The model under review builds one solid part; all positions refer to its coordinate system, in mm. A direction names the side the tool comes from. Coordinates: 2 decimals unless noted, no trailing zeros. Write each loop counter-clockwise with the first axis right and the second up, starting at its lowest first coordinate (ties: lowest second). Pieces come first, ordered by that corner, then holes.
1) For line 1 (X direction, y = -6, z = 101.5); line 2 (Y direction, x = 39, z = 139); line 3 (X direction, y = 52, z = 13), list the stretches that pass through material, from the lowest coordinate up.
2) Mouldability with a two-part tool opening along X and no side actions: class faces 1 (the flat face through (22, 27, 60)), 2 (the flat face through (0, -2, 81)), 3 (the flat face through (-5, 24, 97)) as released by +X, released by -X, zero draft, split by the parting line, or undercut.
3) Add section D-D, the plane x = 30.5. State the section outline as (y, z) points, then the cut area to 3 significant figures.
4) Add section B-B, the plane y = 40. State the section outline as (x, z) points, then the cut area to 3 significant figures.
5) Machinability: for faces 4 (the flat face through (-44, 0, 81)), 5 (the flat face through (5, 24, 97)), 6 (the flat face through (44, 0, 81)), 7 (the flat face through (-26, -7, 81)), which of the approach directions +Z, -Z, +X, -X, +Y, -Y give a long, thin tool a straight path to every point of the face, cutting with its end or side? Answer none if there is none.
6) Add section C-C, the plane z = 146. State the section outline as (x, y) points, then the cut area to 3 significant figures.
7) For P1, Ø9, axis at x = -18.5, y = 19.5, coming from the +Z side; P2, Ø8, axis at x = 31, z = 94.5, coming from the +Y side; P3, Ø6, axis at y = 28, z = 53.5, coming from the +X side, all flat-tipped, find the tip position at first contact; note any pin that passes through.
8) Add section A-A, the plane z = 36. State the section outline as (x, y) points, then the cut area to 3 significant figures.
from build123d import *

# Parameters (mm, degrees)
SKETCH1_W           = 100
SKETCH1_H           = 24
BOSS_EXTRUDE1_DEPTH = 160
SKETCH2_W           = 52
SKETCH2_H           = 10
CUT_EXTRUDE1_DEPTH  = 169.059513268
SKETCH3_W           = 12
SKETCH3_H           = 12
CUT_EXTRUDE2_DEPTH  = 169.059513268
SKETCH4_W           = 77.52732848
SKETCH4_H           = 60
BOSS_EXTRUDE2_DEPTH = 60
FILLET1_RADIUS      = 30
FILLET1_LENGTH      = 77.52732848
SKETCH6_R           = 15
CUT_EXTRUDE3_DEPTH  = 197.629062169
RIB1_REACH          = 184.439
SKETCH7_WALL_W      = 501.963544736
SKETCH7_WALL_H      = 10


with BuildPart() as part:
    # Sketch1 → Boss-Extrude1 (new body)
    with BuildSketch(Plane.XY):
        Rectangle(SKETCH1_W, SKETCH1_H)
    extrude(amount=BOSS_EXTRUDE1_DEPTH)

    # Sketch2 → Cut-Extrude1 (cut, through all)
    with BuildSketch(Plane.XY.offset(160)):
        with Locations((0, -7)):
            Rectangle(SKETCH2_W, SKETCH2_H)
    extrude(amount=-CUT_EXTRUDE1_DEPTH, mode=Mode.SUBTRACT)

    # Sketch3 → Cut-Extrude2 (cut, through all)
    with BuildSketch(Plane.XY.offset(160)):
        with Locations((44.76366424, 6)):
            Rectangle(SKETCH3_W, SKETCH3_H)
    cut_extrude2 = extrude(amount=-CUT_EXTRUDE2_DEPTH, mode=Mode.SUBTRACT)

    # Mirror1: Cut-Extrude2 across plane
    add(cut_extrude2.mirror(Plane(origin=(0, 0, 0), x_dir=(0, 0, 1), z_dir=(1, 0, 0))), mode=Mode.SUBTRACT)

    # Sketch4 → Boss-Extrude2 (add)
    with BuildSketch(Plane(origin=(0, 12, 0), x_dir=(1, 0, 0), z_dir=(0, 1, 0))):
        with Locations((0, -30)):
            Rectangle(SKETCH4_W, SKETCH4_H)
    extrude(amount=BOSS_EXTRUDE2_DEPTH)

    # Fillet1: full round fillet: the end face becomes a half cylinder, R = half its width
    fillet1_face = Plane((0, 72, 30), x_dir=(1, 0, 0), z_dir=(0, 1, 0))  # on the end face: x along it, z out of the body
    fillet1_slab = fillet1_face.offset(-FILLET1_RADIUS / 2) * Box(FILLET1_LENGTH, 2 * FILLET1_RADIUS, FILLET1_RADIUS, mode=Mode.PRIVATE)  # the body's end, R deep
    fillet1_round = Plane((0, 42, 30), x_dir=(0, 1, 0), z_dir=(1, 0, 0)) * Cylinder(FILLET1_RADIUS, FILLET1_LENGTH, mode=Mode.PRIVATE)  # its axis R under the face
    add(fillet1_slab - fillet1_round, mode=Mode.SUBTRACT)

    # Sketch6 → Cut-Extrude3 (cut, through all)
    with BuildSketch(Plane(origin=(38.76366424, 0, 0), x_dir=(0, 0, -1), z_dir=(1, 0, 0))):
        with Locations((-31.347642199, 45.351147576)):
            Circle(SKETCH6_R)
    extrude(amount=-CUT_EXTRUDE3_DEPTH, mode=Mode.SUBTRACT)

    # Sketch7 wall → Rib1 (add, up to next)
    with BuildSketch(Plane(origin=(0, 41.402146272, 99.192634344), x_dir=(0, 0.435311709867, -0.900279798314), z_dir=(0, 0.900279798314, 0.435311709867)), mode=Mode.PRIVATE) as rib1_sk1:
        Rectangle(SKETCH7_WALL_W, SKETCH7_WALL_H)
    rib1_tool1 = extrude(rib1_sk1.sketch, amount=-RIB1_REACH, mode=Mode.PRIVATE) - part.part
    add(rib1_tool1.solids().sort_by_distance((0, 41.402146272, 99.192634344))[0])


solid = part.part
Geometry results:
1. line 1: x = -50 to -26, 26 to 50
1. line 2: y = -12 to 0
1. line 3: x = -38.76 to 38.76
2. face 1: zero draft
2. face 2: undercut
2. face 3: released by -X
3. outline: (-12, 0) - (42, 0) arc R30 ccw to (42, 60) - (12, 60) - (12, 160) - (-12, 160) - close; hole circle Ø30 at (45.35, 31.35)
3. area: 6,350 mm2
4. outline: (-38.76, 0) - (38.76, 0) - (38.76, 17.33) - (-38.76, 17.33) - close; (-38.76, 45.36) - (38.76, 45.36) - (38.76, 60) - (5, 60) - (5, 102.09) - (-5, 102.09) - (-5, 60) - (-38.76, 60) - close
4. area: 2,900 mm2
5. face 4: +Z, -Z, -X, +Y
5. face 5: +Z, +X, +Y
5. face 6: +Z, -Z, +X, +Y
5. face 7: +Z, -Z, -Y
6. outline: (-50, -12) - (-26, -12) - (-26, -2) - (26, -2) - (26, -12) - (50, -12) - (50, 0) - (38.76, 0) - (38.76, 12) - (5, 12) - (5, 18.77) - (-5, 18.77) - (-5, 12) - (-38.76, 12) - (-38.76, 0) - (-50, 0) - close
6. area: 1,680 mm2
7. P1: stops at z = 60
7. P2: stops at y = 12
7. P3: stops at x = 38.76
8. outline: (-50, -12) - (-26, -12) - (-26, -2) - (26, -2) - (26, -12) - (50, -12) - (50, 0) - (38.76, 0) - (38.76, 31.09) - (-38.76, 31.09) - (-38.76, 0) - (-50, 0) - close; (-38.76, 59.61) - (38.76, 59.61) - (38.76, 71.39) - (-38.76, 71.39) - close
8. area: 4,000 mm2
